Model file for the job. Use its own axes, mm. A direction names the side the tool comes from. Give positions to 0.01 mm unless a question says otherwise; leave off trailing zeros. Loops run counter-clockwise (first coordinate to the right, second up) from the corner with the lowest first, then second, coordinate; pieces in that order, holes last. Notation, with made-up numbers: M 51.25,22.5 L 95.25,22.5 A24 ccw 95.25,56.5 Z; hole C 27.5,73.5 d4. An arc over 180 degrees is marked long. Answer in a Markdown table with one row per item.
```python
from build123d import *

# Parameters (mm, degrees)
SKETCH2_W                        = 150
SKETCH2_H                        = 90
SKETCH2_H_2                      = 60
BOSS_EXTRUDE1_DEPTH              = 15
SKETCH3_R                        = 13.005
SKETCH3_R_2                      = 3.01
CUT_EXTRUDE1_DEPTH               = 16
TAP_DRILL_FOR_M8X1_25_TAP2_D     = 6.8
TAP_DRILL_FOR_M8X1_25_TAP2_DEPTH = 10
TAP_DRILL_FOR_M8X1_25_TAP2_TIP   = 2.042926105
TAP_DRILL_FOR_M8X1_25_TAP3_D     = 6.8
TAP_DRILL_FOR_M8X1_25_TAP3_DEPTH = 40
TAP_DRILL_FOR_M8X1_25_TAP3_TIP   = 2.042926105


with BuildPart() as part:
    # Sketch2 → Boss-Extrude1 (new body)
    with BuildSketch(Plane.XY):
        Rectangle(SKETCH2_W, SKETCH2_H)
        with Locations((0, -75)):
            Rectangle(SKETCH2_W, SKETCH2_H_2)
        with BuildLine():
            Line((-75, -105), (75, -105))
            ThreePointArc((75, -105), (0, -136.066017178), (-75, -105))
        make_face()
    extrude(amount=BOSS_EXTRUDE1_DEPTH)

    # Sketch3 → Cut-Extrude1 (cut, through all)
    with BuildSketch(Plane.XY.offset(15)):
        with Locations((0, -85)):
            Circle(SKETCH3_R)
        with Locations((-17, -114.444863729)):
            Circle(SKETCH3_R_2)
        with Locations((0, -119)):
            Circle(SKETCH3_R_2)
    extrude(amount=-CUT_EXTRUDE1_DEPTH, mode=Mode.SUBTRACT)

    # Tap Drill for M8x1.25 Tap2
    with Locations(Plane.XY.offset(15)):
        with Locations((-37.5, -50), (37.5, -50)):
            Hole(TAP_DRILL_FOR_M8X1_25_TAP2_D / 2, depth=TAP_DRILL_FOR_M8X1_25_TAP2_DEPTH)
            with Locations((0, 0, -(TAP_DRILL_FOR_M8X1_25_TAP2_DEPTH + TAP_DRILL_FOR_M8X1_25_TAP2_TIP / 2))):  # 118° drill point
                Cone(0, TAP_DRILL_FOR_M8X1_25_TAP2_D / 2, TAP_DRILL_FOR_M8X1_25_TAP2_TIP, mode=Mode.SUBTRACT)

    # Tap Drill for M8x1.25 Tap3
    with Locations(Plane(origin=(0, 45, 0), x_dir=(1, 0, 0), z_dir=(0, 1, 0))):
        with Locations((-60, -7.5), (60, -7.5)):
            Hole(TAP_DRILL_FOR_M8X1_25_TAP3_D / 2, depth=TAP_DRILL_FOR_M8X1_25_TAP3_DEPTH)
            with Locations((0, 0, -(TAP_DRILL_FOR_M8X1_25_TAP3_DEPTH + TAP_DRILL_FOR_M8X1_25_TAP3_TIP / 2))):  # 118° drill point
                Cone(0, TAP_DRILL_FOR_M8X1_25_TAP3_D / 2, TAP_DRILL_FOR_M8X1_25_TAP3_TIP, mode=Mode.SUBTRACT)


solid = part.part
```
(1) Saw through at A-A, the plane x = -17. Give the cut face in (y, z).
Established:
| item | result |
|---|---|
| outline | M -134.69,0 L -117.45,0 L -117.45,15 L -134.69,15 Z; M -111.43,0 L 45,0 L 45,15 L -111.43,15 Z |
(2) Saw through at B-B, the plane y = -78.5. Give the cut face in (x, z), and give its area (3 significant figures).
Established:
| item | result |
|---|---|
| outline | M -75,0 L -11.26,0 L -11.26,15 L -75,15 Z; M 11.26,0 L 75,0 L 75,15 L 11.26,15 Z |
| area | 1,910 mm2 |
(3) Saw through at C-C, the plane x = 29. Give the cut face in (y, z).
Established:
| item | result |
|---|---|
| outline | M -132.02,0 L 45,0 L 45,15 L -132.02,15 Z |
(4) Saw through at D-D, the plane x = 48. Give the cut face in (y, z).
Established:
| item | result |
|---|---|
| outline | M -124.58,0 L 45,0 L 45,15 L -124.58,15 Z |
(5) Which spindle directions (+Z, -Z, +X, -X, +Y, -Y) get a long thin tool onto all of the face, cutting with end or side? Do faces 4 (the cylindrical face through (-2.8, -97.7, 7.6)), 5 (the cylindrical face through (-63.14, 24.72, 8.8)), 6 (the cylindrical face through (-39.328, -47.133, 9.93)). Say none if no direction does.
Established:
| item | result |
|---|---|
| face 4 | +Z, -Z |
| face 5 | +Y |
| face 6 | +Z |
(6) Flat gauge pin, fed straight in: P1, Ø5.5, axis at x = 37.5, y = -50, coming from the +Z side. Where does the tip first touch, or does it go through?
Established:
| item | result |
|---|---|
| P1 | stops at z = 4.61 |
(7) Mould opens along Z. For faces 1 (the cylindrical face through (56.86, 24.72, 8.8)), 2 (the flat face through (-1, -44, 0)), 3 (the cylindrical face through (1.17, -136.06, 7.4)) say: pulls with the +Z half, pulls with the -Z half, needs draft (parallel to the pull), parting line crosses it, or undercut.
Established:
| item | result |
|---|---|
| face 1 | undercut |
| face 2 | pulls with the -Z half |
| face 3 | needs draft |
(8) Wall check: L1, parallel to X at y = -50, z = 12.75; L2, parallel to Y at x = 0, z = 6.75 (3 decimals); L3, parallel to Z at x = -60, y = 33.5. Give the ranges that are in metal, low to high.
Established:
| item | result |
|---|---|
| L1 | x = -75 to -40.9, -34.1 to 34.1, 40.9 to 75 |
| L2 | y = -136.066 to -122.01, -115.99 to -98.005, -71.995 to 45 |
| L3 | z = 0 to 4.1, 10.9 to 15 |
